Autodesk Inventor part; units mm, degrees
ref_plane "YZ Plane" through (0, 0, 0) normal (1, 0, 0) x (0, 1, 0)
ref_plane "XZ Plane" through (0, 0, 0) normal (0, 1, 0) x (-1, 0, 0)
ref_plane "XY Plane" through (0, 0, 0) normal (0, 0, 1) x (1, 0, 0)
sketch "Sketch2" plane through (0, 0, 0) normal (0, 1, 0) x (-1, 0, 0)
  line L0 (0, 0) -> (-50, 0)
  line L1 (-50, 0) -> (-50, -50)
  line L2 (-50, -50) -> (0, -50)
  line L3 (0, -50) -> (0, 0)
  circle A0 centre (-15, -35) radius 3
  circle A1 centre (-15, -15) radius 3
  line L4 (-15, -35) -> (-15, -50) construction
  line L5 (-15, -15) -> (-15, 0)
  line L6 (-15, -35) -> (0, -35) construction
  line L7 (0, -27) -> (-4, -27)
  line L8 (-4, -23) -> (0, -23)
  line L9 (0, -23) -> (0, -27)
  line L10 (-50, -27) -> (-46, -27)
  line L11 (-46, -23) -> (-50, -23)
  line L12 (-50, -23) -> (-50, -27)
  line L13 (-50, -30) -> (-50, -37)
  line L14 (0, -13) -> (0, -20)
  line L15 (-4, -23) -> (-4, -19)
  line L16 (-4, -19) -> (-46, -19)
  line L17 (-46, -19) -> (-46, -23)
  line L18 (-46, -27) -> (-46, -31)
  line L19 (-46, -31) -> (-4, -31)
  line L20 (-4, -31) -> (-4, -27)
  line L21 (-4, -27) -> (-4, -23)
  line L22 (-46, -27) -> (-46, -23)
  line L23 (-35, 0) -> (-35, -15) construction
  line L24 (-35, -50) -> (-35, -35) construction
  line L25 (-35, -15) -> (-50, -15) construction
  circle A2 centre (-35, -15) radius 3
  circle A3 centre (-35, -35) radius 3
  point P0 (0, -25)
  point P1 (-50, -25)
  point P2 (0, -23)
  dimension "d0" = 50
  dimension "d1" = 6
  dimension "d6" = 4
  dimension "d10" = 7
  dimension "d23" = 15
  dimension "d24" = 4
extrude "Extrusion1" add sketch "Sketch2" along normal blind 10 contours L3 L8 L15 L16 L17 L11 L1 L0 | L10 L18 L19 L20 L7 L3 L2 L1 | L17 L16 L15 L21 L20 L19 L18 L22
extrude "Extrusion2" cut sketch "Sketch2" along normal blind 5 contours L17 L16 L15 L21 L20 L19 L18 L22
fillet "Fillet1" radius 2 2 edges at (4, 5, -25) (46, 5, -25)
equation "\"d0\" = width"
equation "\"d1\" = hole_diameter"
equation "\"d6\" = cabel_shaft_size"
equation "\"d23\" = edge_to_hole"
equation "\"d24\" = cabel_shaft_size"
equation "\"d18\" = plate_thicknes"
equation "\"d20\" = 0.5 * plate_thicknes"
equation "\"width\" = inner_leg_width"
equation "\"cabel_channel_depth\" = 4"
equation "\"plate_thicknes\" = 10"
properties part number "2_inner_leg_top_plate"
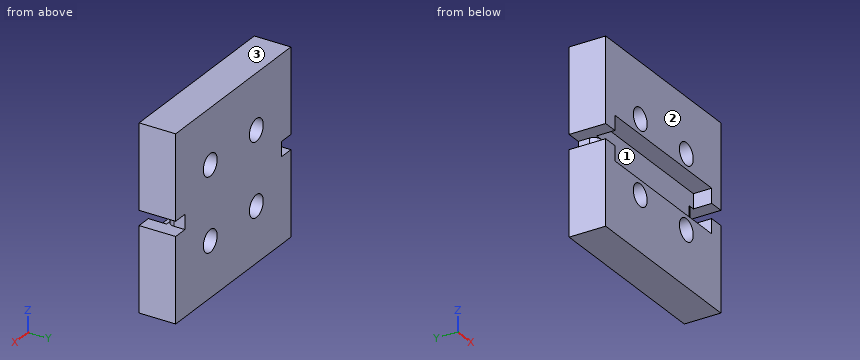
CAD build for the part. Positions are in the model's coordinates, mm. Face numbers are marked on the shaded views. Coordinates: 2 decimals unless noted, no trailing zeros. Write each loop counter-clockwise with the first axis right and the second up, starting at its lowest first coordinate (ties: lowest second). Pieces come first, ordered by that corner, then holes. Notation, with made-up numbers: M 60.25,46.5 L 118.25,46.5 A33 ccw 118.25,75.5 Z; hole C 41,-14 d2. An arc over 180 degrees is marked long. Answer as a JSON object with one key per item and string values. Group by question number.
1) Saw through at D-D (z = -35). Write the cut outline in (x, y).
2) Pin check, flat tip, straight feed: pin 1 Ø0.9 at (y, z) = (8.5, -25) entering from +X. Stop position of the tip, or through.
3) Saw through at B-B (y = 9.25). Write the cut outline in (x, z).
4) Saw through at A-A (y = 1.75). Write the cut outline in (x, z), plus the area to 3 significant figures.
5) Saw through at C-C (x = 15). Write the cut outline in (y, z), plus the area to 3 significant figures.
6) Mould opens along Z. For the marked faces 1, 2 and 3 say: +Z half, -Z half, draft (parallel to the pull), parting line (faces both ways), or undercut.
7) Wall check: line 1 (Z direction, x = 15, y = 2.25); line 2 (Z direction, x = 15, y = 8); line 3 (Z direction, x = 37, y = 2.25). Give the ranges that are in metal, low to high. Write a range as from..to.
Values follow:
{
 "1": {"outline": "M 0,0 L 12,0 L 12,10 L 0,10 Z; M 18,0 L 32,0 L 32,10 L 18,10 Z; M 38,0 L 50,0 L 50,10 L 38,10 Z"},
 "2": {"pin 1": "stops at x = 46"},
 "3": {"outline": "M 0,-50 L 50,-50 L 50,-27 L 46,-27 L 46,-23 L 50,-23 L 50,0 L 0,0 L 0,-23 L 4,-23 L 4,-27 L 0,-27 Z; hole C 15,-35 d6; hole C 15,-15 d6; hole C 35,-35 d6; hole C 35,-15 d6"},
 "4": {"outline": "M 0,-50 L 50,-50 L 50,-27 L 46,-27 L 46,-31 L 4,-31 L 4,-27 L 0,-27 Z; M 0,-23 L 4,-23 L 4,-19 L 46,-19 L 46,-23 L 50,-23 L 50,0 L 0,0 Z; hole C 15,-35 d6; hole C 15,-15 d6; hole C 35,-35 d6; hole C 35,-15 d6", "area": "1,850 mm2"},
 "5": {"outline": "M 0,-50 L 10,-50 L 10,-38 L 0,-38 Z; M 0,-32 L 10,-32 L 10,-18 L 0,-18 L 0,-19 L 5,-19 L 5,-31 L 0,-31 Z; M 0,-12 L 10,-12 L 10,0 L 0,0 Z", "area": "320 mm2"},
 "6": {"face 1": "undercut", "face 2": "draft", "face 3": "+Z half"},
 "7": {"line 1": "z = -50..-38, -32..-31, -19..-18, -12..0", "line 2": "z = -50..-38, -32..-18, -12..0", "line 3": "z = -50..-37.24, -32.76..-31, -19..-17.24, -12.76..0"}
}
